Source: three-view drawing plus pictorial views. Frame: mm from the lowest corner of the part. A direction names the side the tool comes from. Coordinates: 2 decimals unless noted, no trailing zeros. Write each loop counter-clockwise with the first axis right and the second up, starting at its lowest first coordinate (ties: lowest second). Pieces come first, ordered by that corner, then holes. Notation, with made-up numbers: M 25.25,70.5 L 72.25,70.5 A25 ccw 72.25,106.5 Z; hole C 31.5,-24 d3. An arc over 180 degrees is marked long. Write item = value, one per line. Start each with the question number.
Item 1: Ray query, L1, parallel to Z at x = 8.5, y = 6.25; L2, parallel to Y at x = 10, z = 25.5 (1 decimal); L3, parallel to X at y = 4.5, z = 22. Return the intervals inside material, ascending. Write a range as [from, to].
Item 2: Section C-C on x = 7.5. Output: boundary loops of the cut face in (y, z), plus the area to 3 significant figures.
Item 3: Section D-D on y = 12.5. Output: boundary loops of the cut face in (x, z), plus the area to 3 significant figures.
Item 4: Reachability of the marked faces 1, 2 and 3 from +Z, -Z, +X, -X, +Y, -Y: full face, straight path, thin tool, end or side. Return the list, or none.
Item 5: Section B-B on z = 17. Output: boundary loops of the cut face in (x, y).
Item 6: Section A-A on y = 1.5. Output: boundary loops of the cut face in (x, z), plus the area to 3 significant figures.
Item 7: First-contact query: pin 1 Ø1 at (y, z) = (4.5, 1) entering from -X; pin 2 Ø3 at (x, y) = (4.5, 11.5) entering from +Z. Flat tips, straight axial feed; report the tip coordinate or a pass-through.
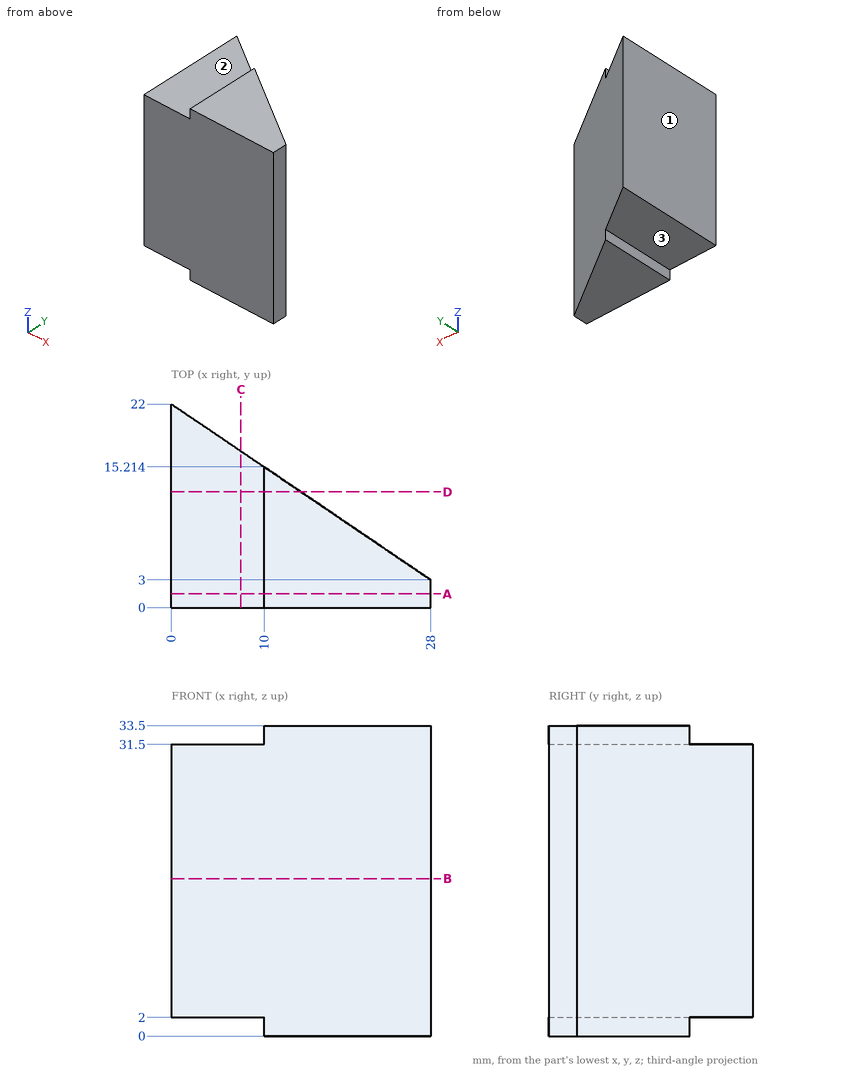
Responses:
q1.L1 = [2, 31.5]
q1.L2 = [0, 15.2]
q1.L3 = [0, 25.79]
q2.outline = M 0,2 L 16.91,2 L 16.91,31.5 L 0,31.5 Z
q2.area = 499 mm²
q3.outline = M 0,2 L 10,2 L 10,0 L 14,0 L 14,33.5 L 10,33.5 L 10,31.5 L 0,31.5 Z
q3.area = 429 mm²
q4.face_1 = +Z, -Z, -X, +Y, -Y
q4.face_2 = +Z, -X, +Y, -Y
q4.face_3 = -Z, -X, +Y, -Y
q5.outline = M 0,0 L 28,0 L 28,3 L 0,22 Z
q6.outline = M 0,2 L 10,2 L 10,0 L 28,0 L 28,33.5 L 10,33.5 L 10,31.5 L 0,31.5 Z
q6.area = 898 mm²
q7.pin_1 = 10
q7.pin_2 = 31.5
